Part print with two shaded views. Sizes in mm from the minimum x, y, z corner. Coordinates: 2 decimals unless noted, no trailing zeros. Order: outer loops, then holes, each group sorted by start corner. A loop starts at its lowest first (then second) coordinate and runs counter-clockwise, first axis right, second up. Notation, with made-up numbers: (46, -18.75) - (66, -18.75) arc R22 ccw to (66, 15.25) - close; hole circle Ø5 at (-16, 1.25). An arc over 180 degrees is marked (long way). Return JSON: item names as keys, results as strings.
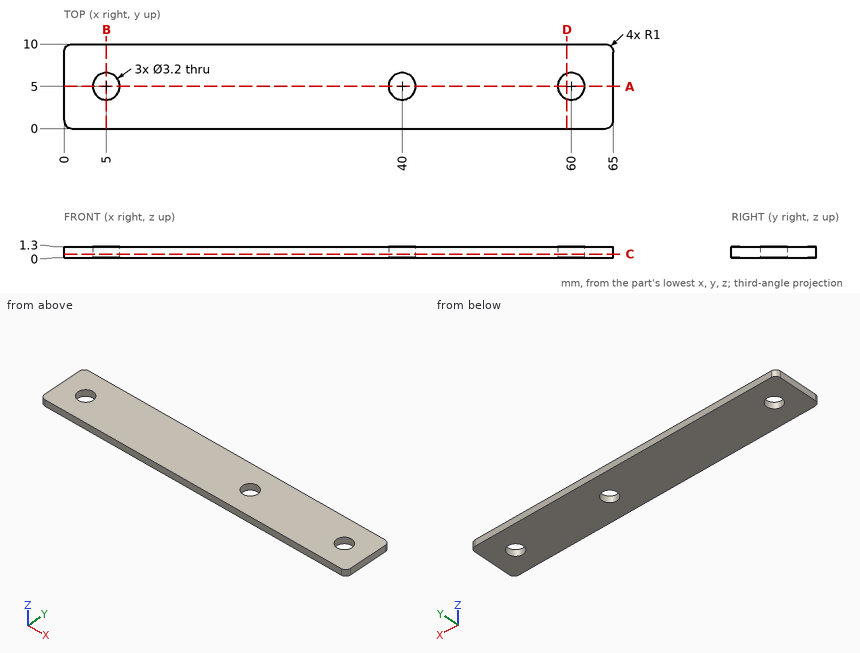
Item 1: Band-saw the part on A-A, the plane y = 5. List the corners of the cut face in (x, z), then the cut area to 3 significant figures.
Findings below:
{"outline": "(0, 0) - (3.4, 0) - (3.4, 1.3) - (0, 1.3) - close; (6.6, 0) - (38.4, 0) - (38.4, 1.3) - (6.6, 1.3) - close; (41.6, 0) - (58.4, 0) - (58.4, 1.3) - (41.6, 1.3) - close; (61.6, 0) - (65, 0) - (65, 1.3) - (61.6, 1.3) - close", "area": "72.0 mm²"}
Item 2: Band-saw the part on D-D, the plane x = 59.5. List the corners of the cut face in (y, z).
Findings below:
{"outline": "(0, 0) - (3.48, 0) - (3.48, 1.3) - (0, 1.3) - close; (6.52, 0) - (10, 0) - (10, 1.3) - (6.52, 1.3) - close"}
Item 3: Band-saw the part on C-C, the plane z = 0.4. List the corners of the cut face in (x, y).
Findings below:
{"outline": "(0, 1) arc R1 ccw to (1, 0) - (64, 0) arc R1 ccw to (65, 1) - (65, 9) arc R1 ccw to (64, 10) - (1, 10) arc R1 ccw to (0, 9) - close; hole circle Ø3.2 at (5, 5); hole circle Ø3.2 at (40, 5); hole circle Ø3.2 at (60, 5)"}
Item 4: Band-saw the part on B-B, the plane x = 5. List the corners of the cut face in (y, z), then the cut area to 3 significant figures.
Findings below:
{"outline": "(0, 0) - (3.4, 0) - (3.4, 1.3) - (0, 1.3) - close; (6.6, 0) - (10, 0) - (10, 1.3) - (6.6, 1.3) - close", "area": "8.84 mm²"}
Item 5: Wall check: L1, parallel to Y at x = 60, z = 0.6; L2, parallel to X at y = 3.75, z = 0.4; L3, parallel to Y at x = 39.5, z = 1.2. Give the ranges that are in metal, low to high. Write a range as [from, to].
Findings below:
{"L1": "y = [0, 3.4], [6.6, 10]", "L2": "x = [0, 4], [6, 39], [41, 59], [61, 65]", "L3": "y = [0, 3.48], [6.52, 10]"}
